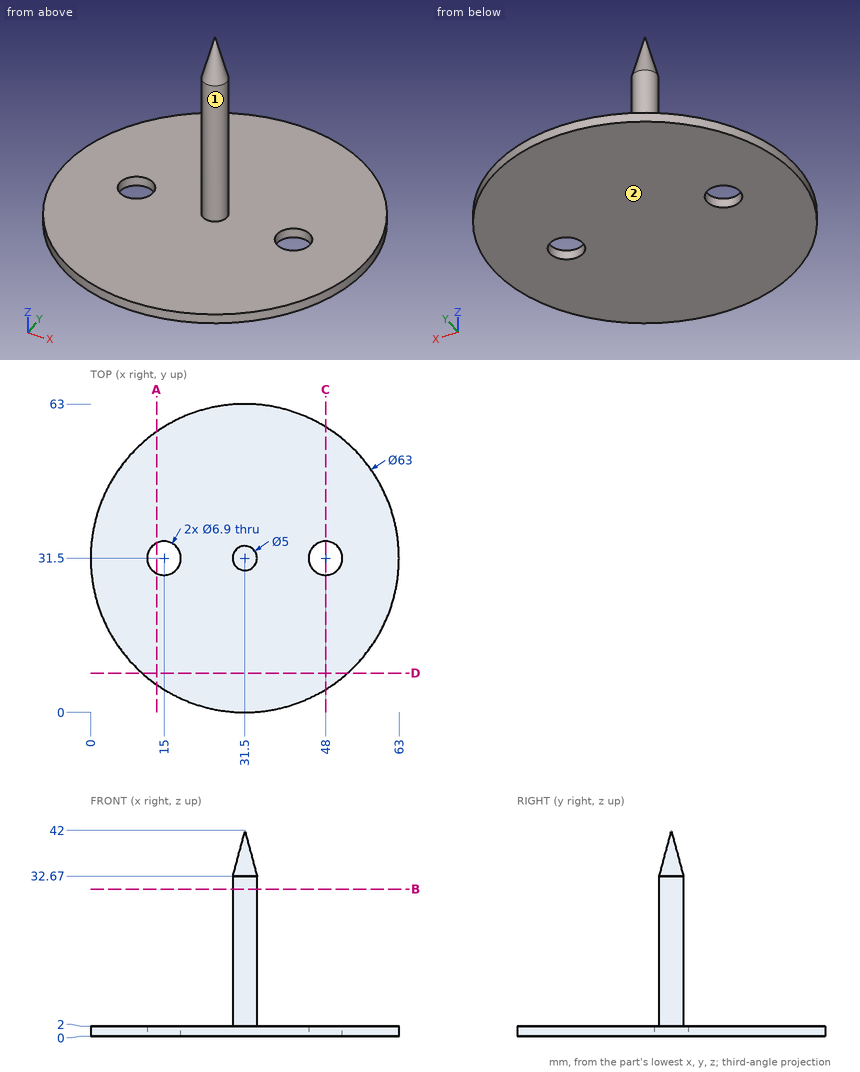
Source: three-view drawing plus pictorial views. Frame: mm from the lowest corner of the part. A direction names the side the tool comes from. Give positions to 0.01 mm unless a question says otherwise; leave off trailing zeros. Order: outer loops, then holes, each group sorted by start corner. A loop starts at its lowest first (then second) coordinate and runs counter-clockwise, first axis right, second up. Notation, with made-up numbers: M 57.5,77.5 L 93.5,77.5 A28 cw 93.5,104.5 Z; hole C 67,-36 d9. An arc over 180 degrees is marked long. One line per question, with ' | ' between items.
1) Access query for the marked faces 1 and 2. Directions: +Z, -Z, +X, -X, +Y, -Y. A direction counts if a zero-diameter tool reaches every point of the face in a straight line with its end or side. Return the directions, or none.
Filled in:
face 1: +Z | face 2: -Z, +X, -X, +Y, -Y
2) Section C-C on x = 48. Output: boundary loops of the cut face in (y, z).
Filled in:
outline: M 4.67,0 L 28.05,0 L 28.05,2 L 4.67,2 Z; M 34.95,0 L 58.33,0 L 58.33,2 L 34.95,2 Z
3) Section B-B on z = 30. Output: boundary loops of the cut face in (x, y).
Filled in:
outline: C 31.5,31.5 d5
4) Ray query, L1, parallel to X at y = 31, z = 1; L2, parallel to Z at x = 12.5, y = 9; L3, parallel to Y at x = 48, z = 1.35. Return the intervals inside material, ascending.
Filled in:
L1: x = 0 to 11.59, 18.41 to 44.59, 51.41 to 63 | L2: z = 0 to 2 | L3: y = 4.67 to 28.05, 34.95 to 58.33
5) Section D-D on y = 8. Output: boundary loops of the cut face in (x, z), and give its area (3 significant figures).
Filled in:
outline: M 10.52,0 L 52.48,0 L 52.48,2 L 10.52,2 Z | area: 83.9 mm2
6) Contact query for flat-ended pins moving along their axis: P1, Ø4, axis at x = 15, y = 31.5, coming from the -Z side; P2, Ø5, axis at x = 25, y = 46.5, coming from the -Z side; P3, Ø9, axis at x = 48, y = 31.5, coming from the +Z side. Output: stop coordinate, or through.
Filled in:
P1: passes through | P2: stops at z = 0 | P3: stops at z = 2
7) Section A-A on x = 13.5. Output: boundary loops of the cut face in (y, z).
Filled in:
outline: M 5.65,0 L 28.39,0 L 28.39,2 L 5.65,2 Z; M 34.61,0 L 57.35,0 L 57.35,2 L 34.61,2 Z
